Part model, mm, in its own coordinate system. Give positions to 0.01 mm unless a question says otherwise; leave off trailing zeros. Write each loop counter-clockwise with the first axis right and the second up, starting at its lowest first coordinate (ties: lowest second). Pieces come first, ordered by that corner, then holes. Notation, with made-up numbers: M 11.25,23 L 68.25,23 A26 ccw 68.25,51 Z; hole C 37,87.25 d5. An arc over 180 degrees is marked long. Use CSV: the item, a comma, the result in double quotes. Start each with the question number.
1. Band-saw the part on B-B, the plane z = -5. Count the separate pieces of the cut face and the enclosed holes in it, then the cut area to 3 significant figures.
2. Mould opens along Z. For faces 1 (the face through (-67.37, 0.79, -23.04)), 2 (the face through (-2, 0.8, -67.9)) say: pulls with the +Z half, pulls with the -Z half, needs draft (parallel to the pull), parting line crosses it, or undercut.
3. Drill centre line: line 1 along Z through (x, y) = (-86, 1.25). Where is it in solid material? Low to high. Write a range as from..to.
4. Band-saw the part on A-A, the plane x = -5. List the corners of the cut face in (y, z).
5. Drop a flat-ended pin along its axis: pin 1 Ø8 at (x, z) = (-64.99, -38.29) entering from -Y. Give the stop position or say it passes through.
Autodesk Inventor part; units mm, degrees
ref_plane "YZ Plane" through (0, 0, 0) normal (1, 0, 0) x (0, 1, 0)
ref_plane "XZ Plane" through (0, 0, 0) normal (0, 1, 0) x (-1, 0, 0)
ref_plane "XY Plane" through (0, 0, 0) normal (0, 0, 1) x (1, 0, 0)
sketch "Sketch1" plane through (0, 0, 0) normal (0, 1, 0) x (-1, 0, 0)
  line L0 (90, 0) -> (90, -70)
  line L1 (90, -70) -> (0, -70)
  line L2 (0, -70) -> (0, 0)
  line L3 (90, 0) -> (0, 0)
  circle A0 centre (85, -5) radius 1.6095
  circle A1 centre (85, -65) radius 1.6095
  circle A2 centre (72.9852, -6.2872) radius 2.5
  circle A3 centre (72.9852, -14.2872) radius 2.5
  circle A4 centre (72.9852, -22.2872) radius 2.5
  circle A5 centre (72.9852, -30.2872) radius 2.5
  circle A6 centre (72.9852, -38.2872) radius 2.5
  circle A7 centre (72.9852, -46.2872) radius 2.5
  circle A8 centre (72.9852, -54.2872) radius 2.5
  circle A9 centre (72.9852, -62.2872) radius 2.5
  circle A10 centre (64.9852, -6.2872) radius 2.5
  circle A11 centre (64.9852, -14.2872) radius 2.5
  circle A12 centre (64.9852, -22.2872) radius 2.5
  circle A13 centre (64.9852, -30.2872) radius 2.5
  circle A14 centre (64.9852, -38.2872) radius 2.5
  circle A15 centre (64.9852, -46.2872) radius 2.5
  circle A16 centre (64.9852, -54.2872) radius 2.5
  circle A17 centre (64.9852, -62.2872) radius 2.5
  circle A18 centre (56.9852, -6.2872) radius 2.5
  circle A19 centre (56.9852, -14.2872) radius 2.5
  circle A20 centre (56.9852, -22.2872) radius 2.5
  circle A21 centre (56.9852, -30.2872) radius 2.5
  circle A22 centre (56.9852, -38.2872) radius 2.5
  circle A23 centre (56.9852, -46.2872) radius 2.5
  circle A24 centre (56.9852, -54.2872) radius 2.5
  circle A25 centre (56.9852, -62.2872) radius 2.5
  circle A26 centre (48.9852, -6.2872) radius 2.5
  circle A27 centre (48.9852, -14.2872) radius 2.5
  circle A28 centre (48.9852, -22.2872) radius 2.5
  circle A29 centre (48.9852, -30.2872) radius 2.5
  circle A30 centre (48.9852, -38.2872) radius 2.5
  circle A31 centre (48.9852, -46.2872) radius 2.5
  circle A32 centre (48.9852, -54.2872) radius 2.5
  circle A33 centre (48.9852, -62.2872) radius 2.5
  circle A34 centre (40.9852, -6.2872) radius 2.5
  circle A35 centre (40.9852, -14.2872) radius 2.5
  circle A36 centre (40.9852, -22.2872) radius 2.5
  circle A37 centre (40.9852, -30.2872) radius 2.5
  circle A38 centre (40.9852, -38.2872) radius 2.5
  circle A39 centre (40.9852, -46.2872) radius 2.5
  circle A40 centre (40.9852, -54.2872) radius 2.5
  circle A41 centre (40.9852, -62.2872) radius 2.5
  circle A42 centre (32.9852, -6.2872) radius 2.5
  circle A43 centre (32.9852, -14.2872) radius 2.5
  circle A44 centre (32.9852, -22.2872) radius 2.5
  circle A45 centre (32.9852, -30.2872) radius 2.5
  circle A46 centre (32.9852, -38.2872) radius 2.5
  circle A47 centre (32.9852, -46.2872) radius 2.5
  circle A48 centre (32.9852, -54.2872) radius 2.5
  circle A49 centre (32.9852, -62.2872) radius 2.5
  circle A50 centre (24.9852, -6.2872) radius 2.5
  circle A51 centre (24.9852, -14.2872) radius 2.5
  circle A52 centre (24.9852, -22.2872) radius 2.5
  circle A53 centre (24.9852, -30.2872) radius 2.5
  circle A54 centre (24.9852, -38.2872) radius 2.5
  circle A55 centre (24.9852, -46.2872) radius 2.5
  circle A56 centre (24.9852, -54.2872) radius 2.5
  circle A57 centre (24.9852, -62.2872) radius 2.5
  circle A58 centre (17.5855, -6.2872) radius 2.5
  circle A59 centre (17.5855, -14.2872) radius 2.5
  circle A60 centre (17.5855, -22.2872) radius 2.5
  circle A61 centre (17.5855, -30.2872) radius 2.5
  circle A62 centre (17.5855, -38.2872) radius 2.5
  circle A63 centre (17.5855, -46.2872) radius 2.5
  circle A64 centre (17.5855, -54.2872) radius 2.5
  circle A65 centre (17.5855, -62.2872) radius 2.5
  circle A66 centre (5, -5) radius 1.6095
  circle A67 centre (5, -65) radius 1.6095
  dimension "d27" = 60
  dimension "d28" = 5
  dimension "d29" = 5
  dimension "d30" = 55.3996
  dimension "d33" = 56
  dimension "d34" = 5
  dimension "d35" = 8
  dimension "d36" = 3
  dimension "d37" = 3
  dimension "d38" = 90
  dimension "d39" = 3.219
extrude "Extrusion1" add sketch "Sketch1" along normal blind 1.6
fillet "Fillet1" radius 7 4 edges at (0, 0.8, 0) (-90, 0.8, 0) (0, 0.8, -70) (-90, 0.8, -70)
properties part number "placa leds" material "PPS Plastic"
Output:
1,separate pieces,"11"
1,enclosed holes,"0"
1,area,"77.9 mm²"
2,face 1,"undercut"
2,face 2,"pulls with the -Z half"
3,line 1,"z = -69.32..-66.26, -63.74..-6.26, -3.74..-0.68"
4,outline,"M 0,-69.71 L 1.6,-69.71 L 1.6,-66.61 L 0,-66.61 Z; M 0,-63.39 L 1.6,-63.39 L 1.6,-6.61 L 0,-6.61 Z; M 0,-3.39 L 1.6,-3.39 L 1.6,-0.29 L 0,-0.29 Z"
5,pin 1,"stops at y = 0"
